```python
from build123d import *

# Parameters (mm, degrees)
SKETCH_2_R          = 1.5
CUT_EXTRUDE_1_DEPTH = 3
CUT_EXTRUDE_START   = -3
SKETCH_3_R          = 1.5
CUT_EXTRUDE_2_DEPTH = 3


with BuildPart() as part:
    # Эскиз1 → Повернуть1 (revolve)
    with BuildSketch(Plane.XY, mode=Mode.PRIVATE) as revolve_1_sk:
        Polygon((0, 0), (9.5, 0), (9.5, 5), (5, 5), (5, 8), (5.9, 8), (5.9, 20), (5, 20), (5, 30), (5.9, 30), (5.9, 45), (0, 45), align=None)
    revolve(revolve_1_sk.sketch.rotate(Axis((0, 14.6467512, 0), (0, -1, 0)), 90), axis=Axis((0, 14.6467512, 0), (0, -1, 0)))

    # Эскиз2 → Вырез-Вытянуть1 (cut)
    with BuildSketch(Plane(origin=(0, 45, 0), x_dir=(1, 0, 0), z_dir=(0, 1, 0))):
        with Locations(Location((0, 0, 0), (0, 0, 270))):
            Circle(SKETCH_2_R)
    extrude(amount=-CUT_EXTRUDE_1_DEPTH, mode=Mode.SUBTRACT)

    # Эскиз3 → Вырез-Вытянуть2 (cut)
    with BuildSketch(Plane(origin=(0, 0, 0), x_dir=(-1, 0, 0), z_dir=(0, -1, 0)).offset(CUT_EXTRUDE_START)):
        with Locations(Location((0, 0, 0), (0, 0, 270))):
            Circle(SKETCH_3_R)
    extrude(amount=CUT_EXTRUDE_2_DEPTH, mode=Mode.SUBTRACT)


solid = part.part
```
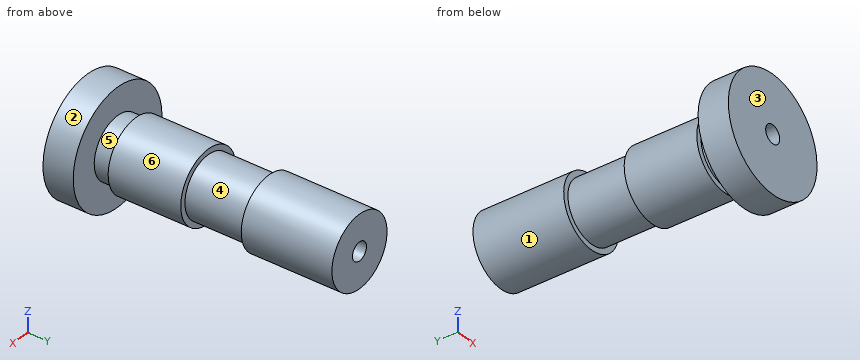
Can you work these out from the model? Positions are in its coordinate system, mm. Face numbers are marked on the shaded views. A direction names the side the tool comes from. Give positions to 0.01 mm unless a question says otherwise; leave off trailing zeros. Loops run counter-clockwise (first coordinate to the right, second up) from the corner with the lowest first, then second, coordinate; pieces in that order, holes last. Notation, with made-up numbers: M 75,65.5 L 92,65.5 A21 ccw 92,79.5 Z; hole C 7,47.25 d3. An arc over 180 degrees is marked long. Answer in a Markdown table with one row per item.
1. Which directions (+Z, -Z, +X, -X, +Y, -Y) give clear straight access to the entire face, cutting with the end or side of a thin tool? Please do the marked faces 1 and 2.
Taken from the geometry:
| item | result |
|---|---|
| face 1 | +Y |
| face 2 | +Y, -Y |
2. If I drill on line 1 along Y through (x, z) = (-4.75, 2.75); line 2 along X through (y, z) = (42.7, 0); line 3 along Y through (x, z) = (6.75, -2.25), over which ranges is the centre line in solid material (lowest first)?
Taken from the geometry:
| item | result |
|---|---|
| line 1 | y = 0 to 5, 8 to 20, 30 to 45 |
| line 2 | x = -5.9 to -1.5, 1.5 to 5.9 |
| line 3 | y = 0 to 5 |
3. Suppose I cut it at A-A on x = 0. Write out the boundary of the cut face in (y, z), plus the area to 3 significant figures.
Taken from the geometry:
| item | result |
|---|---|
| outline | M 0,-9.5 L 5,-9.5 L 5,-5 L 8,-5 L 8,-5.9 L 20,-5.9 L 20,-5 L 30,-5 L 30,-5.9 L 45,-5.9 L 45,-1.5 L 42,-1.5 L 42,1.5 L 45,1.5 L 45,5.9 L 30,5.9 L 30,5 L 20,5 L 20,5.9 L 8,5.9 L 8,5 L 5,5 L 5,9.5 L 0,9.5 L 0,1.5 L 3,1.5 L 3,-1.5 L 0,-1.5 Z |
| area | 526 mm² |
4. For pin 1 Ø3.5 at (x, z) = (0, 0) entering from -Y; pin 2 Ø4 at (y, z) = (35, 6.5) entering from -X; pin 3 Ø6 at (x, y) = (5.5, 30) entering from -Z; pin 4 Ø4 at (x, y) = (4, 14.5) entering from -Z, each with a flat end and sliding along its axis, tell me the tip position at first contact or that it passes through.
Taken from the geometry:
| item | result |
|---|---|
| pin 1 | stops at y = 0 |
| pin 2 | stops at x = -3.82 |
| pin 3 | stops at z = -5.34 |
| pin 4 | stops at z = -5.55 |
5. Thinking about a two-plate mould opening in Y: for the marked faces 3, 4, 5 and 6, which applies, released by +Y, released by -Y, zero draft, split by the parting line, or undercut?
Taken from the geometry:
| item | result |
|---|---|
| face 3 | released by -Y |
| face 4 | undercut |
| face 5 | undercut |
| face 6 | zero draft |
6. Suppose I cut it at C-C on y = 13.5. Write out the boundary of the cut face in (x, z).
Taken from the geometry:
| item | result |
|---|---|
| outline | C 0,0 d11.8 |
7. Suppose I cut it at B-B on z = 0. Write out the boundary of the cut face in (x, y).
Taken from the geometry:
| item | result |
|---|---|
| outline | M -9.5,0 L -1.5,0 L -1.5,3 L 1.5,3 L 1.5,0 L 9.5,0 L 9.5,5 L 5,5 L 5,8 L 5.9,8 L 5.9,20 L 5,20 L 5,30 L 5.9,30 L 5.9,45 L 1.5,45 L 1.5,42 L -1.5,42 L -1.5,45 L -5.9,45 L -5.9,30 L -5,30 L -5,20 L -5.9,20 L -5.9,8 L -5,8 L -5,5 L -9.5,5 Z |
8. Suppose I cut it at D-D on z = -4. Write out the boundary of the cut face in (x, y).
Taken from the geometry:
| item | result |
|---|---|
| outline | M -8.62,0 L 8.62,0 L 8.62,5 L 3,5 L 3,8 L 4.34,8 L 4.34,20 L 3,20 L 3,30 L 4.34,30 L 4.34,45 L -4.34,45 L -4.34,30 L -3,30 L -3,20 L -4.34,20 L -4.34,8 L -3,8 L -3,5 L -8.62,5 Z |
